Source: CAD feature listing. Evaluate the final solid. Frame: model axes, mm. A direction names the side the tool comes from. Give positions to 0.01 mm unless a question says otherwise; leave off trailing zeros. Write each loop counter-clockwise with the first axis right and the second up, starting at its lowest first coordinate (ties: lowest second). Pieces come first, ordered by that corner, then holes. Notation, with made-up numbers: (11, -27) -> (68, -27) arc R5 cw to (68, -19) -> close; hole circle Ø9 at (-12, -17). An arc over 180 degrees is marked (long way). Write item = value, one per line.
Autodesk Inventor part; units mm, degrees
ref_plane "YZ Plane" through (0, 0, 0) normal (1, 0, 0) x (0, 1, 0)
ref_plane "XZ Plane" through (0, 0, 0) normal (0, 1, 0) x (-1, 0, 0)
ref_plane "XY Plane" through (0, 0, 0) normal (0, 0, 1) x (1, 0, 0)
sketch "Sketch4" plane through (0, 0, 0) normal (0, 0, 1) x (1, 0, 0)
  line L0 (0, 0) -> (150, 0)
  line L1 (150, 0) -> (150, 150)
  line L2 (150, 150) -> (0, 150)
  line L3 (0, 150) -> (0, 0)
  dimension "d34" = 150
  dimension "d35" = 150
extrude "Extrusion4" add sketch "Sketch4" along normal blind 10
sketch "Sketch5" plane through (0, 0, 10) normal (0, 0, 1) x (1, 0, 0)
  line L0 (10, 10) -> (140, 10)
  line L1 (140, 10) -> (140, 140)
  line L2 (140, 140) -> (10, 140)
  line L3 (10, 140) -> (10, 10)
  point P0 (0, 0)
  dimension "d38" = 130
  dimension "d39" = 130
extrude "Extrusion5" cut sketch "Sketch5" against normal blind 2
sketch "Sketch6" plane through (0, 0, 0) normal (0, 0, -1) x (-1, 0, 0)
  circle A0 centre (-75, 75) radius 14.35
  circle A1 centre (-75, 75) radius 17.15
  line L0 (-147.5, 2.5) -> (-142.5, 2.5)
  line L1 (-142.5, 2.5) -> (-142.5, 7.5)
  line L2 (-142.5, 7.5) -> (-147.5, 7.5)
  line L3 (-147.5, 7.5) -> (-147.5, 2.5)
  line L4 (-2.5, 2.5) -> (-7.5, 2.5)
  line L5 (-7.5, 2.5) -> (-7.5, 7.5)
  line L6 (-7.5, 7.5) -> (-2.5, 7.5)
  line L7 (-2.5, 7.5) -> (-2.5, 2.5)
  line L8 (-147.5, 147.5) -> (-142.5, 147.5)
  line L9 (-142.5, 147.5) -> (-142.5, 142.5)
  line L10 (-142.5, 142.5) -> (-147.5, 142.5)
  line L11 (-147.5, 142.5) -> (-147.5, 147.5)
  line L12 (-2.5, 147.5) -> (-7.5, 147.5)
  line L13 (-7.5, 147.5) -> (-7.5, 142.5)
  line L14 (-7.5, 142.5) -> (-2.5, 142.5)
  line L15 (-2.5, 142.5) -> (-2.5, 147.5)
  point P0 (0, 0)
  dimension "d42" = 28.7
  dimension "d43" = 34.3
  dimension "d46" = 5
  dimension "d47" = 5
  dimension "d48" = 5
  dimension "d49" = 5
  dimension "d50" = 5
  dimension "d51" = 5
  dimension "d52" = 5
  dimension "d53" = 5
extrude "Extrusion7" cut sketch "Sketch6" against normal blind 5
sketch "Sketch7" plane through (0, 0, 8) normal (0, 0, 1) x (1, 0, 0)
  line L0 (47.5, 102.5) -> (102.5, 102.5)
  line L1 (102.5, 102.5) -> (102.5, 47.5)
  line L2 (102.5, 47.5) -> (47.5, 47.5)
  line L3 (47.5, 47.5) -> (47.5, 102.5)
  point P0 (0, 0)
  dimension "d58" = 55
  dimension "d59" = 55
extrude "Extrusion8" cut sketch "Sketch7" against normal blind 2
sketch "Sketch8" plane through (0, 0, 10) normal (0, 0, 1) x (1, 0, 0)
  line L0 (0, 0) -> (150, 0)
  line L1 (150, 0) -> (150, 150)
  line L2 (150, 150) -> (0, 150)
  line L3 (0, 150) -> (0, 0)
  line L4 (37.5, 112.5) -> (112.5, 112.5)
  line L5 (112.5, 112.5) -> (112.5, 37.5)
  line L6 (112.5, 37.5) -> (37.5, 37.5)
  line L7 (37.5, 37.5) -> (37.5, 112.5)
  dimension "d62" = 150
  dimension "d63" = 150
  dimension "d64" = 75
  dimension "d65" = 75
extrude "Extrusion9" cut sketch "Sketch8" against normal blind 10
sketch "Sketch9" plane through (0, 0, 6) normal (0, 0, 1) x (1, 0, 0)
  line L0 (47.5, 47.5) -> (47.5, 102.5)
  line L1 (47.5, 47.5) -> (102.5, 47.5)
  line L2 (102.5, 47.5) -> (102.5, 102.5)
  line L3 (102.5, 102.5) -> (47.5, 102.5)
  line L4 (47.5, 102.5) -> (47.5, 47.5)
  point P0 (0, 0)
  dimension "d68" = 55
  dimension "d69" = 55
extrude "Extrusion10" add sketch "Sketch9" along normal blind 2
sketch "Sketch10" plane through (0, 0, 8) normal (0, 0, 1) x (1, 0, 0)
  line L0 (37.5, 37.5) -> (112.5, 37.5)
  line L1 (112.5, 37.5) -> (112.5, 112.5)
  line L2 (37.5, 37.5) -> (112.5, 37.5)
  line L3 (112.5, 37.5) -> (112.5, 112.5)
  line L4 (112.5, 112.5) -> (37.5, 112.5)
  line L5 (37.5, 112.5) -> (37.5, 37.5)
  point P0 (0, 0)
  dimension "d72" = 75
  dimension "d73" = 75
extrude "Extrusion11" add sketch "Sketch10" along normal blind 5
sketch "Sketch11" plane through (0, 0, 13) normal (0, 0, 1) x (1, 0, 0)
  line L0 (47.5, 47.5) -> (102.5, 47.5)
  line L1 (102.5, 47.5) -> (102.5, 102.5)
  line L2 (102.5, 102.5) -> (47.5, 102.5)
  line L3 (47.5, 102.5) -> (47.5, 47.5)
  point P0 (0, 0)
  dimension "d76" = 55
  dimension "d77" = 55
extrude "Extrusion12" cut sketch "Sketch11" against normal blind 2
sketch "Sketch12" plane through (0, 0, 11) normal (0, 0, 1) x (1, 0, 0)
  circle A0 centre (75, 75) radius 14.35
  circle A1 centre (75, 75) radius 17.15
  point P0 (0, 0)
properties part number "Elbow_Parallel_Joint"
1) Cut plane B-B (y = 75). Return the cut outline in (x, z).
Computed:
outline = (37.5, 0) -> (57.85, 0) -> (57.85, 5) -> (60.65, 5) -> (60.65, 0) -> (89.35, 0) -> (89.35, 5) -> (92.15, 5) -> (92.15, 0) -> (112.5, 0) -> (112.5, 13) -> (102.5, 13) -> (102.5, 11) -> (47.5, 11) -> (47.5, 13) -> (37.5, 13) -> close
2) Material intervals for L1, parallel to Y at x = 75, z = 1.4; L2, parallel to Y at x = 90.5, z = 12.75; L3, parallel to Y at x = 65, z = 4.75, sorted ascending.
Computed:
L1 = 37.5 to 57.85, 60.65 to 89.35, 92.15 to 112.5
L2 = 37.5 to 47.5, 102.5 to 112.5
L3 = 37.5 to 61.07, 64.71 to 85.29, 88.93 to 112.5
3) Cut plane D-D (x = 97). Return the cut outline in (y, z).
Computed:
outline = (37.5, 0) -> (112.5, 0) -> (112.5, 13) -> (102.5, 13) -> (102.5, 11) -> (47.5, 11) -> (47.5, 13) -> (37.5, 13) -> close
4) Access query for faces 4 (the flat face through (79, 61, 5)), 5 (the flat face through (75, 47.5, 12)), 6 (the flat face through (76, 112.5, 6)). Directions: +Z, -Z, +X, -X, +Y, -Y. A direction counts if a zero-diameter tool reaches every point of the face in a straight line with its end or side. Return the directions, or none.
Computed:
face_4 = -Z
face_5 = +Z
face_6 = +Z, -Z, +X, -X, +Y
5) Cut plane A-A (z = 2). Return the cut outline in (x, y), then the cut area to 3 significant figures.
Computed:
outline = (37.5, 37.5) -> (112.5, 37.5) -> (112.5, 112.5) -> (37.5, 112.5) -> close; circle Ø28.7 at (75, 75); hole circle Ø34.3 at (75, 75)
area = 5,350 mm²
6) Draft query along Y for faces 1 (the flat face through (112.5, 74, 6)), 2 (the cylindrical face through (89.336, 75.631, 2.465)), 3 (the flat face through (74, 37.5, 6)). Return one class per face: pulls with the +Y half, pulls with the -Y half, needs draft (parallel to the pull), parting line crosses it, or undercut.
Computed:
face_1 = needs draft
face_2 = undercut
face_3 = pulls with the -Y half
